Here's how the part is built. I have some questions about the finished solid (model axes, mm). Face numbers are marked on the shaded views. Round coordinates to 2 decimals unless told otherwise and drop trailing zeros. Loops run counter-clockwise (first coordinate to the right, second up) from the corner with the lowest first, then second, coordinate; pieces in that order, holes last. Notation, with made-up numbers: M -9.75,-15.75 L 3.25,-15.75 A31 cw 3.25,22.25 Z; hole C -27.75,67 d6. An arc over 180 degrees is marked long. Use a Markdown table: item, result.
```python
from build123d import *

# Parameters (mm, degrees)
F0_R     = 3.175
F1_DEPTH = 3.048
F2_DEPTH = 25.4
F3_DEPTH = 3.048


with BuildPart() as f1:
    # F0 (on Front) → F1 (new body)
    with BuildSketch(Plane.XZ):
        with BuildLine():
            ThreePointArc((-9.450293, 115.490625), (-0.596483, 104.793695), (9.525, 114.3))
            ThreePointArc((9.525, 114.3), (9.506305, 114.896483), (9.450293, 115.490625))
            ThreePointArc((9.450293, 115.490625), (0, 123.825), (-9.450293, 115.490625))
        make_face()
        with Locations((0, 114.3)):
            Circle(F0_R, mode=Mode.SUBTRACT)
        with BuildLine():
            ThreePointArc((9.450293, 115.490625), (9.506305, 114.896483), (9.525, 114.3))
            ThreePointArc((9.525, 114.3), (-0.596483, 104.793695), (-9.450293, 115.490625))
            Line((-9.450293, 115.490625), (-15.750488, 65.484375))
            ThreePointArc((-15.750488, 65.484375), (0, 79.375), (15.750488, 65.484375))
            Line((15.750488, 65.484375), (9.450293, 115.490625))
        make_face()
        with Locations((-3.175, 100.0252)):
            Circle(F0_R, mode=Mode.SUBTRACT)
        with BuildLine():
            ThreePointArc((15.875, 63.5), (15.843841, 64.494139), (15.750488, 65.484375))
            ThreePointArc((15.750488, 65.484375), (0, 79.375), (-15.750488, 65.484375))
            ThreePointArc((-15.750488, 65.484375), (-15.873744, 63.699705), (-15.795426, 61.9125))
            ThreePointArc((-15.795426, 61.9125), (-0.199705, 47.626256), (15.750488, 61.515625))
            ThreePointArc((15.750488, 61.515625), (15.843841, 62.505861), (15.875, 63.5))
        make_face()
        with Locations((0, 63.5)):
            Circle(F0_R, mode=Mode.SUBTRACT)
        with BuildLine():
            ThreePointArc((15.750488, 61.515625), (-0.199705, 47.626256), (-15.795426, 61.9125))
            Line((-15.795426, 61.9125), (-9.477255, -0.9525))
            ThreePointArc((-9.477255, -0.9525), (-7.063929, 6.389564), (0, 9.525))
            ThreePointArc((0, 9.525), (0.253535, 9.521625), (0.506891, 9.511503))
            ThreePointArc((0.506891, 9.511503), (6.912082, 6.553529), (9.525, 0))
            ThreePointArc((9.525, 0), (6.912082, -6.553529), (0.506891, -9.511503))
            Line((0.506891, -9.511503), (35.885598, -8.569463))
            ThreePointArc((35.885598, -8.569463), (27.084916, 0), (35.885598, 8.569463))
            Line((35.885598, 8.569463), (17.942799, 9.047231))
            ThreePointArc((17.942799, 9.047231), (12.122303, 11.815881), (10.266572, 17.988389))
            Line((10.266572, 17.988389), (15.750488, 61.515625))
        make_face()
        with BuildLine():
            ThreePointArc((0, 9.525), (-7.063929, 6.389564), (-9.477255, -0.9525))
            ThreePointArc((-9.477255, -0.9525), (-6.389564, -7.063929), (0, -9.525))
            Line((0, -9.525), (0.506891, -9.511503))
            ThreePointArc((0.506891, -9.511503), (6.912082, -6.553529), (9.525, 0))
            ThreePointArc((9.525, 0), (6.912082, 6.553529), (0.506891, 9.511503))
            Line((0.506891, 9.511503), (0, 9.525))
        make_face()
        Circle(F0_R, mode=Mode.SUBTRACT)
        with BuildLine():
            Line((0.506891, -9.511503), (0, -9.525))
            ThreePointArc((0, -9.525), (0.253535, -9.521625), (0.506891, -9.511503))
        make_face()
        with BuildLine():
            ThreePointArc((44.229916, 0), (41.799234, 5.980454), (35.885598, 8.569463))
            ThreePointArc((35.885598, 8.569463), (27.084916, 0), (35.885598, -8.569463))
            ThreePointArc((35.885598, -8.569463), (41.799234, -5.980454), (44.229916, 0))
        make_face()
        with Locations((35.657416, 0)):
            Circle(F0_R, mode=Mode.SUBTRACT)
    extrude(amount=F1_DEPTH)

    # F0 (on Front) → F2 (join)
    with BuildSketch(Plane.XZ):
        with BuildLine():
            ThreePointArc((-9.450293, 115.490625), (-0.596483, 104.793695), (9.525, 114.3))
            ThreePointArc((9.525, 114.3), (9.506305, 114.896483), (9.450293, 115.490625))
            ThreePointArc((9.450293, 115.490625), (0, 123.825), (-9.450293, 115.490625))
        make_face()
        with Locations((0, 114.3)):
            Circle(F0_R, mode=Mode.SUBTRACT)
        with BuildLine():
            ThreePointArc((9.450293, 115.490625), (9.506305, 114.896483), (9.525, 114.3))
            ThreePointArc((9.525, 114.3), (-0.596483, 104.793695), (-9.450293, 115.490625))
            Line((-9.450293, 115.490625), (-15.750488, 65.484375))
            ThreePointArc((-15.750488, 65.484375), (0, 79.375), (15.750488, 65.484375))
            Line((15.750488, 65.484375), (9.450293, 115.490625))
        make_face()
        with Locations((-3.175, 100.0252)):
            Circle(F0_R, mode=Mode.SUBTRACT)
        with BuildLine():
            ThreePointArc((15.875, 63.5), (15.843841, 64.494139), (15.750488, 65.484375))
            ThreePointArc((15.750488, 65.484375), (0, 79.375), (-15.750488, 65.484375))
            ThreePointArc((-15.750488, 65.484375), (-15.873744, 63.699705), (-15.795426, 61.9125))
            ThreePointArc((-15.795426, 61.9125), (-0.199705, 47.626256), (15.750488, 61.515625))
            ThreePointArc((15.750488, 61.515625), (15.843841, 62.505861), (15.875, 63.5))
        make_face()
        with Locations((0, 63.5)):
            Circle(F0_R, mode=Mode.SUBTRACT)
        with BuildLine():
            ThreePointArc((15.750488, 61.515625), (-0.199705, 47.626256), (-15.795426, 61.9125))
            Line((-15.795426, 61.9125), (-9.477255, -0.9525))
            ThreePointArc((-9.477255, -0.9525), (-7.063929, 6.389564), (0, 9.525))
            ThreePointArc((0, 9.525), (0.253535, 9.521625), (0.506891, 9.511503))
            ThreePointArc((0.506891, 9.511503), (6.912082, 6.553529), (9.525, 0))
            ThreePointArc((9.525, 0), (6.912082, -6.553529), (0.506891, -9.511503))
            Line((0.506891, -9.511503), (35.885598, -8.569463))
            ThreePointArc((35.885598, -8.569463), (27.084916, 0), (35.885598, 8.569463))
            Line((35.885598, 8.569463), (17.942799, 9.047231))
            ThreePointArc((17.942799, 9.047231), (12.122303, 11.815881), (10.266572, 17.988389))
            Line((10.266572, 17.988389), (15.750488, 61.515625))
        make_face()
        with BuildLine():
            ThreePointArc((0, 9.525), (-7.063929, 6.389564), (-9.477255, -0.9525))
            ThreePointArc((-9.477255, -0.9525), (-6.389564, -7.063929), (0, -9.525))
            Line((0, -9.525), (0.506891, -9.511503))
            ThreePointArc((0.506891, -9.511503), (6.912082, -6.553529), (9.525, 0))
            ThreePointArc((9.525, 0), (6.912082, 6.553529), (0.506891, 9.511503))
            Line((0.506891, 9.511503), (0, 9.525))
        make_face()
        Circle(F0_R, mode=Mode.SUBTRACT)
        with BuildLine():
            Line((0.506891, -9.511503), (0, -9.525))
            ThreePointArc((0, -9.525), (0.253535, -9.521625), (0.506891, -9.511503))
        make_face()
        with BuildLine():
            ThreePointArc((44.229916, 0), (41.799234, 5.980454), (35.885598, 8.569463))
            ThreePointArc((35.885598, 8.569463), (27.084916, 0), (35.885598, -8.569463))
            ThreePointArc((35.885598, -8.569463), (41.799234, -5.980454), (44.229916, 0))
        make_face()
        with Locations((35.657416, 0)):
            Circle(F0_R, mode=Mode.SUBTRACT)
    extrude(amount=F2_DEPTH)

    # F0 (on Front) → F3 (join)
    with BuildSketch(Plane.XZ):
        with BuildLine():
            ThreePointArc((-9.450293, 115.490625), (-0.596483, 104.793695), (9.525, 114.3))
            ThreePointArc((9.525, 114.3), (9.506305, 114.896483), (9.450293, 115.490625))
            ThreePointArc((9.450293, 115.490625), (0, 123.825), (-9.450293, 115.490625))
        make_face()
        with Locations((0, 114.3)):
            Circle(F0_R, mode=Mode.SUBTRACT)
        with BuildLine():
            ThreePointArc((9.450293, 115.490625), (9.506305, 114.896483), (9.525, 114.3))
            ThreePointArc((9.525, 114.3), (-0.596483, 104.793695), (-9.450293, 115.490625))
            Line((-9.450293, 115.490625), (-15.750488, 65.484375))
            ThreePointArc((-15.750488, 65.484375), (0, 79.375), (15.750488, 65.484375))
            Line((15.750488, 65.484375), (9.450293, 115.490625))
        make_face()
        with Locations((-3.175, 100.0252)):
            Circle(F0_R, mode=Mode.SUBTRACT)
        with BuildLine():
            ThreePointArc((15.875, 63.5), (15.843841, 64.494139), (15.750488, 65.484375))
            ThreePointArc((15.750488, 65.484375), (0, 79.375), (-15.750488, 65.484375))
            ThreePointArc((-15.750488, 65.484375), (-15.873744, 63.699705), (-15.795426, 61.9125))
            ThreePointArc((-15.795426, 61.9125), (-0.199705, 47.626256), (15.750488, 61.515625))
            ThreePointArc((15.750488, 61.515625), (15.843841, 62.505861), (15.875, 63.5))
        make_face()
        with Locations((0, 63.5)):
            Circle(F0_R, mode=Mode.SUBTRACT)
        with BuildLine():
            ThreePointArc((15.750488, 61.515625), (-0.199705, 47.626256), (-15.795426, 61.9125))
            Line((-15.795426, 61.9125), (-9.477255, -0.9525))
            ThreePointArc((-9.477255, -0.9525), (-7.063929, 6.389564), (0, 9.525))
            ThreePointArc((0, 9.525), (0.253535, 9.521625), (0.506891, 9.511503))
            ThreePointArc((0.506891, 9.511503), (6.912082, 6.553529), (9.525, 0))
            ThreePointArc((9.525, 0), (6.912082, -6.553529), (0.506891, -9.511503))
            Line((0.506891, -9.511503), (35.885598, -8.569463))
            ThreePointArc((35.885598, -8.569463), (27.084916, 0), (35.885598, 8.569463))
            Line((35.885598, 8.569463), (17.942799, 9.047231))
            ThreePointArc((17.942799, 9.047231), (12.122303, 11.815881), (10.266572, 17.988389))
            Line((10.266572, 17.988389), (15.750488, 61.515625))
        make_face()
        with BuildLine():
            ThreePointArc((0, 9.525), (-7.063929, 6.389564), (-9.477255, -0.9525))
            ThreePointArc((-9.477255, -0.9525), (-6.389564, -7.063929), (0, -9.525))
            Line((0, -9.525), (0.506891, -9.511503))
            ThreePointArc((0.506891, -9.511503), (6.912082, -6.553529), (9.525, 0))
            ThreePointArc((9.525, 0), (6.912082, 6.553529), (0.506891, 9.511503))
            Line((0.506891, 9.511503), (0, 9.525))
        make_face()
        Circle(F0_R, mode=Mode.SUBTRACT)
        with BuildLine():
            Line((0.506891, -9.511503), (0, -9.525))
            ThreePointArc((0, -9.525), (0.253535, -9.521625), (0.506891, -9.511503))
        make_face()
        with BuildLine():
            ThreePointArc((44.229916, 0), (41.799234, 5.980454), (35.885598, 8.569463))
            ThreePointArc((35.885598, 8.569463), (27.084916, 0), (35.885598, -8.569463))
            ThreePointArc((35.885598, -8.569463), (41.799234, -5.980454), (44.229916, 0))
        make_face()
        with Locations((35.657416, 0)):
            Circle(F0_R, mode=Mode.SUBTRACT)
    extrude(amount=F3_DEPTH)


solid = f1.part
```
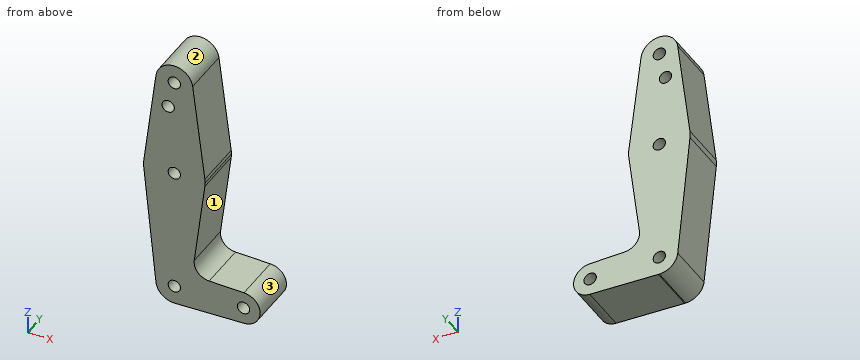
Q1. Imagine slicing it at C-C, the plane z = 114.3. Please give me the cut outline in (x, y) (3 decimals), then the cut area to 3 significant figures.
Return value:
| item | result |
|---|---|
| outline | M -9.6,-25.4 L -3.175,-25.4 L -3.175,0 L -9.6,0 Z; M 3.175,-25.4 L 9.6,-25.4 L 9.6,0 L 3.175,0 Z |
| area | 326 mm^2 |
Q2. Imagine slicing it at D-D, the plane x = 31. Please give me the cut outline in (y, z).
Return value:
| item | result |
|---|---|
| outline | M -25.4,-8.7 L 0,-8.7 L 0,8.7 L -25.4,8.7 Z |
Q3. I need wall thicknesses on line 1 (Z direction, x = -0.5, y = -3.75); line 2 (X direction, y = -5, z = 98.5); line 3 (Z direction, x = 6.5, y = -9.5). Which ranges of each line are inside material? Lowest first, please. Write a range as from..to.
Return value:
| item | result |
|---|---|
| line 1 | z = -9.51..-3.14, 3.14..60.36, 66.64..98.31, 101.74..111.16, 117.44..123.81 |
| line 2 | x = -11.59..-5.96, -0.39..11.59 |
| line 3 | z = -9.35..121.26 |
Q4. Imagine slicing it at A-A, the plane x = -1.5. Please give me the cut outline in (y, z), then the cut area to 3 significant figures.
Return value:
| item | result |
|---|---|
| outline | M -25.4,-9.41 L 0,-9.41 L 0,-2.8 L -25.4,-2.8 Z; M -25.4,2.8 L 0,2.8 L 0,60.7 L -25.4,60.7 Z; M -25.4,66.3 L 0,66.3 L 0,97.33 L -25.4,97.33 Z; M -25.4,102.72 L 0,102.72 L 0,111.5 L -25.4,111.5 Z; M -25.4,117.1 L 0,117.1 L 0,123.71 L -25.4,123.71 Z |
| area | 2,820 mm^2 |
Q5. We'd pull the mould along Z, two halves only. Please class the marked faces 1, 2 and 3: pulls with the +Z half, pulls with the -Z half, needs draft (parallel to the pull), parting line crosses it, or undercut.
Return value:
| item | result |
|---|---|
| face 1 | undercut |
| face 2 | pulls with the +Z half |
| face 3 | parting line crosses it |
Q6. Will these pins go through, and if not, where does the flat tip stop? P1, Ø6, axis at x = -7, y = -20, coming from the +Z side; P2, Ø4, axis at y = -7.5, z = 32.5, coming from the -X side; P3, Ø3, axis at x = 21, y = -9, coming from the -Z side.
Return value:
| item | result |
|---|---|
| P1 | stops at z = 122.94 |
| P2 | stops at x = -13.04 |
| P3 | stops at z = -9.01 |
